Here's how the part is built. I have some questions about the finished solid (model axes, mm). Face numbers are marked on the shaded views. A direction names the side the tool comes from. Coordinates: 2 decimals unless noted, no trailing zeros. Write each loop counter-clockwise with the first axis right and the second up, starting at its lowest first coordinate (ties: lowest second). Pieces come first, ordered by that corner, then holes. Notation, with made-up numbers: (62, -38) -> (72, -38) arc R26 cw to (72, -3) -> close; hole circle Ø2 at (43, 83). An arc over 180 degrees is marked (long way). Put each result on its own line as item: value.
Autodesk Inventor part; units mm, degrees
ref_plane "YZ Plane" through (0, 0, 0) normal (1, 0, 0) x (0, 1, 0)
ref_plane "XZ Plane" through (0, 0, 0) normal (0, 1, 0) x (-1, 0, 0)
ref_plane "XY Plane" through (0, 0, 0) normal (0, 0, 1) x (1, 0, 0)
sketch "Sketch1" plane through (0, 0, 0) normal (0, 0, 1) x (1, 0, 0)
  arc A0 (0, 9.75) -> (0, -9.75) centre (0, 0) ccw
  line L0 (0, 9.75) -> (25, 9.75)
  line L1 (25, -9.75) -> (0, -9.75)
  line L2 (25, 9.75) -> (25, 29.75)
  line L3 (25, 29.75) -> (32, 29.75)
  line L4 (32, 29.75) -> (32, 9.75)
  line L5 (32, 9.75) -> (32, -9.75)
  line L6 (32, -9.75) -> (32, -29.75)
  line L7 (32, -29.75) -> (25, -29.75)
  line L8 (25, -29.75) -> (25, -9.75)
  dimension "d0" = 19.5
  dimension "d1" = 25
  dimension "d4" = 20
  dimension "d5" = 7
  dimension "d6" = 20
  dimension "d7" = 59.5
  dimension "d8" = 20
extrude "Extrusion1" add sketch "Sketch1" along normal blind 4.6
properties part number "Air Restricter 1.1"
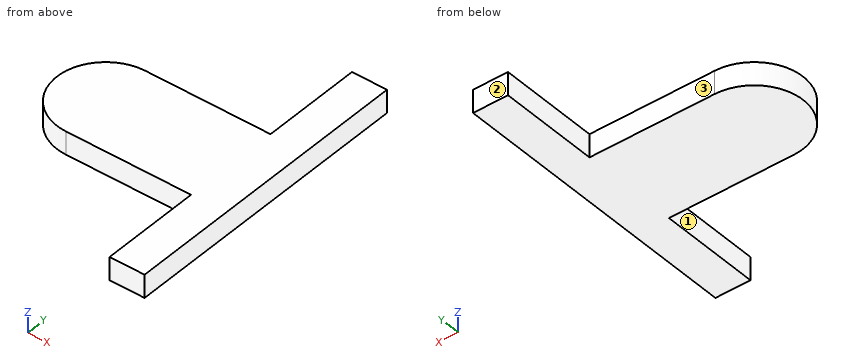
Item 1: Imagine slicing it at B-B on x = 13. Write out the boundary of the cut face in (y, z), then the cut area to 3 significant figures.
Output:
outline: (-9.75, 0) -> (9.75, 0) -> (9.75, 4.6) -> (-9.75, 4.6) -> close
area: 89.7 mm²
Item 2: Which directions (+Z, -Z, +X, -X, +Y, -Y) give clear straight access to the entire face, cutting with the end or side of a thin tool? Please do the marked faces 1, 2 and 3.
Output:
face 1: +Z, -Z, -X, -Y
face 2: +Z, -Z, +X, -X, +Y
face 3: +Z, -Z, -X, +Y
Item 3: For P1, Ø1.4, axis at x = 11.5, z = 2, coming from the +Y side; P2, Ø8, axis at x = 1.5, y = -13.5, coming from the +Z side; P3, Ø1.5, axis at y = 17, z = 2, coming from the -X side, each with a flat end and sliding along its axis, tell me the tip position at first contact or that it passes through.
Output:
P1: stops at y = 9.75
P2: stops at z = 4.6
P3: stops at x = 25
Item 4: Please list where these lines run through material, in increasing order: line 1 along Y through (x, z) = (17, 0.9); line 2 along X through (y, z) = (-25.5, 3.7); line 3 along X through (y, z) = (1.5, 4.05). Write a range as from..to.
Output:
line 1: y = -9.75..9.75
line 2: x = 25..32
line 3: x = -9.63..32
Item 5: Imagine slicing it at A-A on z = 1.55. Write out the boundary of the cut face in (x, y).
Output:
outline: (0, -9.75) -> (25, -9.75) -> (25, -29.75) -> (32, -29.75) -> (32, 29.75) -> (25, 29.75) -> (25, 9.75) -> (0, 9.75) arc R9.75 ccw to start
Item 6: Imagine slicing it at C-C on y = 25. Write out the boundary of the cut face in (x, z), then the cut area to 3 significant figures.
Output:
outline: (25, 0) -> (32, 0) -> (32, 4.6) -> (25, 4.6) -> close
area: 32.2 mm²
